Can you work these out from the model? Positions are in its coordinate system, mm. A direction names the side the tool comes from. Give positions to 0.01 mm unless a question says otherwise; leave off trailing zeros. Loops run counter-clockwise (first coordinate to the right, second up) from the corner with the lowest first, then second, coordinate; pieces in that order, holes last. Notation, with made-up numbers: M -18,-6 L -8,-6 A24 ccw -8,28 Z; hole C 25,7.25 d3. An arc over 180 degrees is marked long. Put each result on its own line as item: value. Start each with the question number.
1) If we mould it in two halves opening along X, with no side actions, what happens to faces 1 (the flat face through (2, 3.175, 3)), 2 (the flat face through (28.659, 8.417, 0.981)), 3 (the flat face through (-0.39, 8.74, 5.55))? For each: +X half, -X half, draft (parallel to the pull), parting line (faces both ways), or undercut.
2) Imagine slicing it at C-C (z = 12.25). Write out the boundary of the cut face in (x, y), then the cut area to 3 significant figures.
3) Please list where these lines run through material, in increasing order: line 1 along Z through (x, y) = (3, 5.5); line 2 along X through (y, z) = (0, 2.25) (3 decimals). Write a range as from..to.
4) For P1, Ø4.5, axis at x = -7, y = 0.5, coming from the +Z side (3 decimals); P2, Ø10, axis at x = 2, z = 13, coming from the -Y side; P3, Ø5, axis at x = -12, y = -7.5, coming from the +Z side; P4, Ø4, axis at y = -3.5, z = 17, coming from the +X side, each with a flat end and sliding along its axis, tell me the tip position at first contact or that it passes through.
5) For faces 4 (the cylindrical face through (13.668, 0.106, 12.22)), 5 (the flat face through (9.525, 0, 3)), 6 (the flat face through (-16, 0, 19.05)), which set-ups out of +Z, -Z, +X, -X, +Y, -Y let a thin tool reach every point of the face, with its end or its side?
6) Imagine slicing it at D-D (y = -4.75). Write out the boundary of the cut face in (x, z), then the cut area to 3 significant figures.
from build123d import *

# Parameters (mm, degrees)
F0_W     = 59.490514
F0_H     = 19.05
F1_DEPTH = 6.35
F2_R     = 2.413
F3_DEPTH = 12.7
F4_W     = 19.05
F4_H     = 6.35
F5_DEPTH = 3.175
F6_W     = 12.7
F6_H     = 6.35
F7_DEPTH = 19.051
F8_SIZE  = 0.79375
F9_SIZE  = 1.5875
F10_SIZE = 0.79375


with BuildPart() as f1:
    # F0 (on Top) → F1 (new body)
    with BuildSketch(Plane.XY):
        Rectangle(F0_W, F0_H)
    extrude(amount=F1_DEPTH)

    # F2 (on face) → F3 (join)
    with BuildSketch(Plane.XY.offset(6.35)):
        with Locations((-16.0782, 0)):
            Circle(F2_R)
        with Locations((16.0782, 0)):
            Circle(F2_R)
    extrude(amount=F3_DEPTH)

    # F4 (on face) → F5 (cut)
    with BuildSketch(Plane.XY.offset(6.35)):
        Rectangle(F4_W, F4_H)
    extrude(amount=-F5_DEPTH, mode=Mode.SUBTRACT)

    # F6 (on face) → F7 (cut, through all)
    with BuildSketch(Plane(origin=(0, 0, 0), x_dir=(1, 0, 0), z_dir=(0, 0, -1))):
        with Locations((3.175, 0)):
            Rectangle(F6_W, F6_H)
    extrude(amount=-F7_DEPTH, mode=Mode.SUBTRACT)

    # F8
    f8_edges = [f1.edges().sort_by_distance(p)[0] for p in [
        (-3.175, 0, 3.175),
        (-3.175, 0, 0),
        (0, 3.175, 6.35),
        (9.525, 0, 6.35),
        (0, -3.175, 6.35),
        (-9.525, 0, 6.35),
    ]]
    chamfer(f8_edges, length=F8_SIZE)

    # F9
    f9_edges = [f1.edges().sort_by_distance(p)[0] for p in [
        (-29.745257, -9.525, 3.175),
        (29.745257, -9.525, 3.175),
        (0, -9.525, 0),
        (0, -9.525, 6.35),
        (29.745257, 9.525, 3.175),
        (29.745257, 0, 0),
        (29.745257, 0, 6.35),
        (-29.745257, 9.525, 3.175),
        (0, 9.525, 0),
        (0, 9.525, 6.35),
        (-29.745257, 0, 0),
        (-29.745257, 0, 6.35),
    ]]
    chamfer(f9_edges, length=F9_SIZE)

    # F10
    f10_edges = [f1.edges().sort_by_distance(p)[0] for p in [
        (13.6652, 0, 19.05),
        (-18.4912, 0, 19.05),
    ]]
    chamfer(f10_edges, length=F10_SIZE)


solid = f1.part
Recorded:
1. face 1: undercut
1. face 2: +X half
1. face 3: draft
2. outline: C -16.08,0 d4.83; C 16.08,0 d4.83
2. area: 36.6 mm²
3. line 1: 0..6.35
3. line 2: -29.745..-3.175, 9.525..29.745
4. P1: z = 3.175
4. P2: through
4. P3: z = 6.35
4. P4: x = 17.97
5. face 4: +Z
5. face 5: +Z, -Z
5. face 6: +Z, +X, -X, +Y, -Y
6. outline: M -29.75,1.59 L -28.16,0 L 28.16,0 L 29.75,1.59 L 29.75,4.76 L 28.16,6.35 L -28.16,6.35 L -29.75,4.76 Z
6. area: 373 mm²
